Geometry: final body of the model. Coordinates: model frame, mm. Face numbers are marked on the shaded views. A direction names the side the tool comes from. Give positions to 0.01 mm unless a question says otherwise; leave off trailing zeros. Write each loop counter-clockwise with the first axis right and the second up, starting at its lowest first coordinate (ties: lowest second). Pieces come first, ordered by that corner, then holes. Notation, with made-up numbers: M 88,-4.75 L 107,-4.75 A9 cw 107,1.25 Z; hole C -14,71 d11. An arc over 180 degrees is marked long. Use a Markdown table: item, result. Add a question column.
1) Set-up query: the marked faces 1, 2 and 3. Return all of +Z, -Z, +X, -X, +Y, -Y with unobstructed straight access to the full face (end or side cutting, diameter ignored); none if empty.
2) Section D-D on z = 2.25. Return the cut outline in (x, y), then the cut area to 3 significant figures.
3) Pin query (flat end, axial travel): pin 1 (1 mm diameter, centred on x = 69, y = -88.5, fed in from -Z); pin 2 (3.5 mm diameter, centred on x = 73.66, y = -95.64, fed in from -Z); pin 3 (0.8 mm diameter, centred on x = 78.5, z = -1, fed in from -Y); pin 4 (1.7 mm diameter, centred on y = -75, z = -1, fed in from +X). Return the tip coordinate at first contact, or that it passes through.
4) Section B-B on y = -80.5. Return the cut outline in (x, z), then the cut area to 3 significant figures.
5) Line query: line 1 (Y direction, x = 73.66, z = 2.2); line 2 (X direction, y = -77, z = 1.75); line 3 (X direction, y = -81.25, z = 5). Output: solid intervals per line, ascending.
6) Section A-A on x = 73.66. Return the cut outline in (y, z), then the cut area to 3 significant figures.
7) Section C-C on z = -2. Return the cut outline in (x, y).
8) Draft query along X for the marked faces 4, 5 and 6. Return one class per face: +X half, -X half, draft (parallel to the pull), parting line (faces both ways), or undercut.
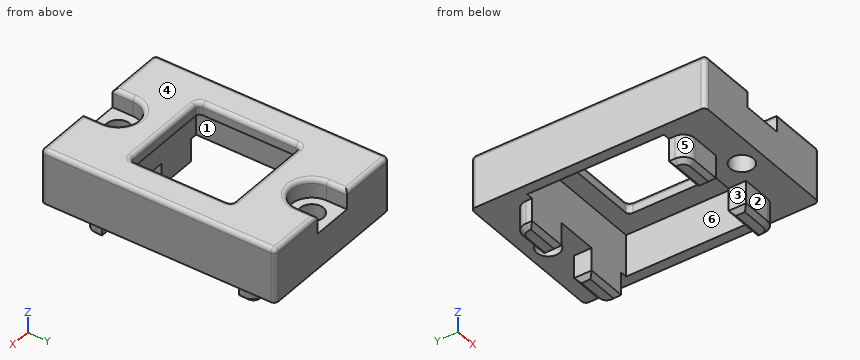
```python
from build123d import *

# Parameters (mm, degrees)
SKETCH1_W                                      = 18.415
SKETCH1_H                                      = 27.432
BOSS_EXTRUDE1_DEPTH                            = 6.35
SKETCH2_W                                      = 11.1125
SKETCH2_H                                      = 11.90625
CUT_EXTRUDE1_DEPTH                             = 7.35
SHELL1_T                                       = -1
BOSS_EXTRUDE2_REACH                            = 8.35
SKETCH5_W                                      = 5.7752
SKETCH5_H                                      = 5.7752
CBORE_FOR_2_SOCKET_HEAD_CAP_SCREW2_D           = 2.7051
CBORE_FOR_2_SOCKET_HEAD_CAP_SCREW2_CBORE_D     = 4.7625
CBORE_FOR_2_SOCKET_HEAD_CAP_SCREW2_CBORE_DEPTH = 2.1844
CUT_EXTRUDE2_DEPTH                             = 4.9276
SKETCH7_W                                      = 11.1125
SKETCH7_H                                      = 11.90625
BOSS_EXTRUDE4_DEPTH                            = 0.4224
SKETCH8_W                                      = 4.7625
SKETCH8_H                                      = 2.3876
CUT_EXTRUDE3_DEPTH                             = 2.1844
FILLET1_R                                      = 0.508
BOSS_EXTRUDE5_REACH                            = 8.35
SKETCH10_W                                     = 16
SKETCH10_H                                     = 16
BOSS_EXTRUDE6_DEPTH                            = 3.175
CHAMFER1_SIZE                                  = 0.508


with BuildPart() as part:
    # Sketch1 → Boss-Extrude1 (new body)
    with BuildSketch(Plane.XY):
        with Locations((73.66, -84.3122297)):
            Rectangle(SKETCH1_W, SKETCH1_H)
    extrude(amount=BOSS_EXTRUDE1_DEPTH)

    # Sketch2 → Cut-Extrude1 (cut, through all)
    with BuildSketch(Plane.XY.offset(6.35)):
        with Locations((73.66, -84.3122297)):
            Rectangle(SKETCH2_W, SKETCH2_H)
    extrude(amount=-CUT_EXTRUDE1_DEPTH, mode=Mode.SUBTRACT)

    # Shell1
    shell1_openings = [part.faces().sort_by_distance(p)[0] for p in [
        (73.66, -90.2653547, 3.175),
        (68.10375, -84.3122297, 3.175),
        (73.66, -78.3591047, 3.175),
        (79.21625, -84.3122297, 3.175),
        (73.66, -84.3122297, 0),
    ]]
    offset(amount=SHELL1_T, openings=shell1_openings, kind=Kind.INTERSECTION)

    # Sketch5 → Boss-Extrude2 (add, up to next)
    with BuildSketch(Plane(origin=(0, 0, 0), x_dir=(-1, 0, 0), z_dir=(0, 0, -1)), mode=Mode.PRIVATE) as boss_extrude2_sk1:
        with Locations((-73.66, -73.4838297)):
            Rectangle(SKETCH5_W, SKETCH5_H)
    boss_extrude2_tool1 = extrude(boss_extrude2_sk1.sketch, amount=-BOSS_EXTRUDE2_REACH, mode=Mode.PRIVATE) - part.part
    add(boss_extrude2_tool1.solids().sort_by_distance((73.66, -73.48383, 0))[0])
    # Sketch5 → Boss-Extrude2 (add, up to next)
    with BuildSketch(Plane(origin=(0, 0, 0), x_dir=(-1, 0, 0), z_dir=(0, 0, -1)), mode=Mode.PRIVATE) as boss_extrude2_sk2:
        with Locations((-73.66, -95.1406297)):
            Rectangle(SKETCH5_W, SKETCH5_H)
    boss_extrude2_tool2 = extrude(boss_extrude2_sk2.sketch, amount=-BOSS_EXTRUDE2_REACH, mode=Mode.PRIVATE) - part.part
    add(boss_extrude2_tool2.solids().sort_by_distance((73.66, -95.14063, 0))[0])

    # CBORE for #2 Socket Head Cap Screw2 (through all)
    with Locations(Plane.XY.offset(6.35)):
        with Locations((73.66, -95.6406297), (73.66, -72.9838297)):
            CounterBoreHole(CBORE_FOR_2_SOCKET_HEAD_CAP_SCREW2_D / 2, CBORE_FOR_2_SOCKET_HEAD_CAP_SCREW2_CBORE_D / 2, CBORE_FOR_2_SOCKET_HEAD_CAP_SCREW2_CBORE_DEPTH)

    # Sketch6 → Cut-Extrude2 (cut)
    with BuildSketch(Plane(origin=(0, 0, 0), x_dir=(-1, 0, 0), z_dir=(0, 0, -1))):
        with BuildLine():
            Line((-76.5476, -95.6406297), (-76.8016, -95.6406297))
            Line((-76.8016, -95.6406297), (-76.8016, -92.2530297))
            Line((-76.8016, -92.2530297), (-70.5184, -92.2530297))
            Line((-70.5184, -92.2530297), (-70.5184, -95.6406297))
            Line((-70.5184, -95.6406297), (-70.7724, -95.6406297))
            ThreePointArc((-70.7724, -95.6406297), (-73.66, -92.7530297), (-76.5476, -95.6406297))
        make_face()
        with BuildLine():
            Line((-76.8016, -72.9838297), (-76.8016, -76.3714297))
            Line((-76.8016, -76.3714297), (-70.5184, -76.3714297))
            Line((-70.5184, -76.3714297), (-70.5184, -72.9838297))
            Line((-70.5184, -72.9838297), (-70.7724, -72.9838297))
            ThreePointArc((-70.7724, -72.9838297), (-73.66, -75.8714297), (-76.5476, -72.9838297))
            Line((-76.5476, -72.9838297), (-76.8016, -72.9838297))
        make_face()
    extrude(amount=-CUT_EXTRUDE2_DEPTH, mode=Mode.SUBTRACT)

    # Sketch7 → Boss-Extrude4 (add)
    with BuildSketch(Plane(origin=(0, 0, 5.35), x_dir=(-1, 0, 0), z_dir=(0, 0, -1))):
        Polygon((-70.7724, -76.3714297), (-76.5476, -76.3714297), (-76.5476, -71.5962297), (-81.8675, -71.5962297), (-81.8675, -97.0282297), (-76.5476, -97.0282297), (-76.5476, -92.2530297), (-70.7724, -92.2530297), (-70.7724, -97.0282297), (-65.4525, -97.0282297), (-65.4525, -71.5962297), (-70.7724, -71.5962297), align=None)
        with Locations((-73.66, -84.3122297)):
            Rectangle(SKETCH7_W, SKETCH7_H, mode=Mode.SUBTRACT)
    extrude(amount=BOSS_EXTRUDE4_DEPTH)

    # Sketch8 → Cut-Extrude3 (cut)
    with BuildSketch(Plane.XY.offset(6.35)):
        with Locations((73.66, -96.8344297)):
            Rectangle(SKETCH8_W, SKETCH8_H)
        with Locations((73.66, -71.7900297)):
            Rectangle(SKETCH8_W, SKETCH8_H)
    extrude(amount=-CUT_EXTRUDE3_DEPTH, mode=Mode.SUBTRACT)

    # Fillet1
    fillet1_edges = [part.edges().sort_by_distance(p)[0] for p in [
        (79.454375, -70.5962297, 6.35),
        (73.66, -93.2593797, 6.35),
        (64.4525, -84.3122297, 6.35),
        (79.21625, -90.2653547, 5.6388),
        (68.10375, -90.2653547, 5.6388),
        (68.10375, -78.3591047, 5.6388),
        (79.21625, -78.3591047, 5.6388),
        (73.66, -90.2653547, 6.35),
        (79.21625, -84.3122297, 6.35),
        (73.66, -78.3591047, 6.35),
        (68.10375, -84.3122297, 6.35),
        (79.454375, -98.0282297, 6.35),
        (76.04125, -96.8344297, 6.35),
        (71.27875, -96.8344297, 6.35),
        (73.66, -75.3650797, 6.35),
        (67.865625, -70.5962297, 6.35),
        (71.27875, -71.7900297, 6.35),
        (76.04125, -71.7900297, 6.35),
        (67.865625, -98.0282297, 6.35),
        (82.8675, -84.3122297, 6.35),
        (64.4525, -98.0282297, 3.175),
        (64.4525, -70.5962297, 3.175),
        (82.8675, -70.5962297, 3.175),
        (82.8675, -98.0282297, 3.175),
    ]]
    fillet(fillet1_edges, radius=FILLET1_R)

    # Sketch10 → Boss-Extrude5 (add, up to next)
    with BuildSketch(Plane(origin=(0, 0, 0), x_dir=(-1, 0, 0), z_dir=(0, 0, -1)), mode=Mode.PRIVATE) as boss_extrude5_sk1:
        with BuildLine():
            Line((-76.5476, -97.0282297), (-76.5476, -95.6406297))
            ThreePointArc((-76.5476, -95.6406297), (-73.66, -92.7530297), (-70.7724, -95.6406297))
            Line((-70.7724, -95.6406297), (-70.7724, -97.0282297))
            Line((-70.7724, -97.0282297), (-65.4525, -97.0282297))
            Line((-65.4525, -97.0282297), (-65.4525, -71.5962297))
            Line((-65.4525, -71.5962297), (-70.7724, -71.5962297))
            Line((-70.7724, -71.5962297), (-70.7724, -72.9838297))
            ThreePointArc((-70.7724, -72.9838297), (-73.66, -75.8714297), (-76.5476, -72.9838297))
            Line((-76.5476, -72.9838297), (-76.5476, -71.5962297))
            Line((-76.5476, -71.5962297), (-81.8675, -71.5962297))
            Line((-81.8675, -71.5962297), (-81.8675, -97.0282297))
            Line((-81.8675, -97.0282297), (-76.5476, -97.0282297))
        make_face()
        with Locations((-73.66, -84.3122297)):
            Rectangle(SKETCH10_W, SKETCH10_H, mode=Mode.SUBTRACT)
    boss_extrude5_tool1 = extrude(boss_extrude5_sk1.sketch, amount=-BOSS_EXTRUDE5_REACH, mode=Mode.PRIVATE) - part.part
    add(boss_extrude5_tool1.solids().sort_by_distance((76.850294, -72.29003, 0))[0])

    # Sketch11 → Boss-Extrude6 (add)
    with BuildSketch(Plane(origin=(0, 0, 0), x_dir=(-1, 0, 0), z_dir=(0, 0, -1))):
        with BuildLine():
            Line((-66.461462743, -92.3122297), (-66.461462743, -93.0447297))
            ThreePointArc((-66.461462743, -93.0447297), (-66.85203585, -93.987656593), (-67.794962743, -94.3782297))
            Line((-67.794962743, -94.3782297), (-71.223962743, -94.3782297))
            Line((-71.223962743, -94.3782297), (-71.223962743, -92.3122297))
            Line((-71.223962743, -92.3122297), (-66.461462743, -92.3122297))
        make_face()
        with BuildLine():
            Line((-76.096037257, -92.3122297), (-80.858537257, -92.3122297))
            Line((-80.858537257, -92.3122297), (-80.858537257, -93.0447297))
            ThreePointArc((-80.858537257, -93.0447297), (-80.46796415, -93.987656593), (-79.525037257, -94.3782297))
            Line((-79.525037257, -94.3782297), (-76.096037257, -94.3782297))
            Line((-76.096037257, -94.3782297), (-76.096037257, -92.3122297))
        make_face()
        with BuildLine():
            Line((-80.858537257, -76.3122297), (-80.858537257, -75.5797297))
            ThreePointArc((-80.858537257, -75.5797297), (-80.46796415, -74.636802807), (-79.525037257, -74.2462297))
            Line((-79.525037257, -74.2462297), (-76.096037257, -74.2462297))
            Line((-76.096037257, -74.2462297), (-76.096037257, -76.3122297))
            Line((-76.096037257, -76.3122297), (-80.858537257, -76.3122297))
        make_face()
        with BuildLine():
            Line((-71.223962743, -76.3122297), (-66.461462743, -76.3122297))
            Line((-66.461462743, -76.3122297), (-66.461462743, -75.5797297))
            ThreePointArc((-66.461462743, -75.5797297), (-66.85203585, -74.636802807), (-67.794962743, -74.2462297))
            Line((-67.794962743, -74.2462297), (-71.223962743, -74.2462297))
            Line((-71.223962743, -74.2462297), (-71.223962743, -76.3122297))
        make_face()
    extrude(amount=BOSS_EXTRUDE6_DEPTH)

    # Chamfer1
    chamfer1_edges = [part.edges().sort_by_distance(p)[0] for p in [
        (68.842712743, -92.3122297, -3.175),
        (71.223962743, -93.3452297, -3.175),
        (69.509462743, -94.3782297, -3.175),
        (66.85203585, -93.987656593, -3.175),
        (66.461462743, -92.6784797, -3.175),
        (80.858537257, -92.6784797, -3.175),
        (80.46796415, -93.987656593, -3.175),
        (77.810537257, -94.3782297, -3.175),
        (76.096037257, -93.3452297, -3.175),
        (78.477287257, -92.3122297, -3.175),
        (80.46796415, -74.636802807, -3.175),
        (80.858537257, -75.9459797, -3.175),
        (78.477287257, -76.3122297, -3.175),
        (76.096037257, -75.2792297, -3.175),
        (77.810537257, -74.2462297, -3.175),
        (66.461462743, -75.9459797, -3.175),
        (66.85203585, -74.636802807, -3.175),
        (69.509462743, -74.2462297, -3.175),
        (71.223962743, -75.2792297, -3.175),
        (68.842712743, -76.3122297, -3.175),
    ]]
    chamfer(chamfer1_edges, length=CHAMFER1_SIZE)


solid = part.part
```
Found:
| question | item | result |
|---|---|---|
| 1 | face 1 | -Z |
| 1 | face 2 | -Z, +X, -X, -Y |
| 1 | face 3 | -Z, +Y, -Y |
| 2 | outline | M 64.45,-97.52 A0.51 ccw 64.96,-98.03 L 82.36,-98.03 A0.51 ccw 82.87,-97.52 L 82.87,-71.1 A0.51 ccw 82.36,-70.6 L 64.96,-70.6 A0.51 ccw 64.45,-71.1 Z; hole M 65.66,-92.31 L 81.66,-92.31 L 81.66,-76.31 L 65.66,-76.31 Z; hole C 73.66,-95.64 d2.71; hole C 73.66,-72.98 d2.71 |
| 2 | area | 237 mm² |
| 3 | pin 1 | through |
| 3 | pin 2 | z = 0 |
| 3 | pin 3 | y = -94.38 |
| 3 | pin 4 | x = 80.86 |
| 4 | outline | M 64.45,0 L 65.66,0 L 65.66,4.93 L 68.1,4.93 L 68.1,5.84 A0.51 ccw 67.6,6.35 L 64.96,6.35 A0.51 ccw 64.45,5.84 Z; M 79.22,4.93 L 81.66,4.93 L 81.66,0 L 82.87,0 L 82.87,5.84 A0.51 ccw 82.36,6.35 L 79.72,6.35 A0.51 ccw 79.22,5.84 Z |
| 4 | area | 22.1 mm² |
| 5 | line 1 | -98.03 to -96.99, -94.29 to -92.31, -76.31 to -74.34, -71.63 to -70.6 |
| 5 | line 2 | 64.45 to 65.66, 81.66 to 82.87 |
| 5 | line 3 | 64.45 to 68.1, 79.22 to 82.87 |
| 6 | outline | M -98.03,0 L -96.99,0 L -96.99,4.17 L -98.03,4.17 Z; M -94.29,0 L -92.31,0 L -92.31,4.93 L -90.27,4.93 L -90.27,5.84 A0.51 ccw -90.77,6.35 L -92.75,6.35 A0.51 ccw -93.26,5.84 L -93.26,4.17 L -94.29,4.17 Z; M -78.36,4.93 L -76.31,4.93 L -76.31,0 L -74.34,0 L -74.34,4.17 L -75.37,4.17 L -75.37,5.84 A0.51 ccw -75.87,6.35 L -77.85,6.35 A0.51 ccw -78.36,5.84 Z; M -71.63,0 L -70.6,0 L -70.6,4.17 L -71.63,4.17 Z |
| 6 | area | 34.8 mm² |
| 7 | outline | M 66.46,-93.04 A1.33 ccw 67.79,-94.38 L 71.22,-94.38 L 71.22,-92.31 L 66.46,-92.31 Z; M 66.46,-76.31 L 71.22,-76.31 L 71.22,-74.25 L 67.79,-74.25 A1.33 ccw 66.46,-75.58 Z; M 76.1,-94.38 L 79.53,-94.38 A1.33 ccw 80.86,-93.04 L 80.86,-92.31 L 76.1,-92.31 Z; M 76.1,-76.31 L 80.86,-76.31 L 80.86,-75.58 A1.33 ccw 79.53,-74.25 L 76.1,-74.25 Z |
| 8 | face 4 | draft |
| 8 | face 5 | -X half |
| 8 | face 6 | undercut |
